from build123d import *

# Parameters (mm, degrees)
BOSS_EXTRUDE1_DEPTH      = 25
CUT_EXTRUDE4_START       = 8.5
CUT_EXTRUDE4_DEPTH       = 8
SKETCH10_R               = 4.2
CUT_EXTRUDE6_DEPTH       = 122.590026426
SKETCH11_W               = 24
SKETCH11_H               = 24.52
BOSS_EXTRUDE2_DEPTH      = 10
CUT_EXTRUDE7_DEPTH       = 122.590026426
CUT_EXTRUDE8_START       = 5.5
SKETCH14_W               = 24
SKETCH14_H               = 20.52
CUT_EXTRUDE8_DEPTH       = 2
SKETCH22_R               = 12.6
CUT_EXTRUDE16_DEPTH      = 122.590026426
SKETCH24_W               = 17.5
SKETCH24_H               = 12
BOSS_EXTRUDE3_DEPTH      = 25
FILLET6_R                = 15
FILLET7_R                = 1
SKETCH25_R               = 3
CUT_EXTRUDE18_DEPTH      = 25
SKETCH26_W               = 2.5
SKETCH26_H               = 20
CUT_EXTRUDE19_DEPTH      = 25
SHELL14_START            = 9.25
SHELL14_DEPTH            = 1.5
SHELL14_START_2          = 3
SHELL14_2_DEPTH          = 19
SHELL14_3_OUTLINE_R      = 9.2
SHELL14_3_DEPTH          = 0.5
SHELL14_START_3          = 21.5
SHELL14_4_OUTLINE_R      = 9.2
SHELL14_4_DEPTH          = 0.5
SHELL14_START_4          = 8
SHELL14_5_DEPTH          = 2.75
SHELL14_START_5          = 19.25
SHELL14_6_DEPTH          = 1.5
SKETCH27_W               = 17.72
SKETCH27_H               = 18.5
CUT_EXTRUDE20_DEPTH      = 10
SKETCH28_W               = 14
SKETCH28_H               = 35
CUT_EXTRUDE21_DEPTH      = 3
SKETCH29_W               = 14
SKETCH29_H               = 35
CUT_EXTRUDE22_DEPTH      = 3
FILLET8_R                = 4
FILLET9_R                = 4
FILLET10_R               = 1
CUT_EXTRUDE23_DEPTH      = 132.116752851
CUT_EXTRUDE23_DEPTH_BACK = 132.116752851
SKETCH32_W               = 24
SKETCH32_H               = 0.7
CUT_EXTRUDE24_DEPTH      = 132.116752851
FILLET11_R               = 3
BOSS_EXTRUDE4_REACH      = 133.117
SKETCH33_W               = 28
SKETCH33_H               = 2


with BuildPart() as part:
    # Sketch1 → Boss-Extrude1 (new body)
    with BuildSketch(Plane.XY):
        with BuildLine():
            Line((30, 0), (30, 75))
            ThreePointArc((30, 75), (15, 113.093476939), (0, 75))
            Line((0, 75), (0, 0))
            ThreePointArc((0, 0), (15, -15), (30, 0))
        make_face()
    extrude(amount=BOSS_EXTRUDE1_DEPTH)

    # Sketch9 → Cut-Extrude4 (cut)
    with BuildSketch(Plane.XY.offset(CUT_EXTRUDE4_START)):
        with BuildLine():
            Line((7.015640289, 0), (0, -3.844579475))
            Line((0, -3.844579475), (0, -19.136394538))
            Line((0, -19.136394538), (30, -19.136394538))
            Line((30, -19.136394538), (30, -3.844579475))
            Line((30, -3.844579475), (22.984359711, 0))
            ThreePointArc((22.984359711, 0), (15, 8.5), (7.015640289, 0))
        make_face()
    extrude(amount=CUT_EXTRUDE4_DEPTH, mode=Mode.SUBTRACT)

    # Sketch10 → Cut-Extrude6 (cut, through all)
    with BuildSketch(Plane.XY):
        with Locations(Location((15, 0.5, 0), (0, 0, 180))):
            Circle(SKETCH10_R)
    extrude(amount=CUT_EXTRUDE6_DEPTH, mode=Mode.SUBTRACT)

    # Sketch11 → Boss-Extrude2 (add)
    with BuildSketch(Plane(origin=(0, 0, 0), x_dir=(-1, 0, 0), z_dir=(0, 0, -1))):
        with Locations((-15, 32.26)):
            Rectangle(SKETCH11_W, SKETCH11_H)
    extrude(amount=BOSS_EXTRUDE2_DEPTH)

    # Sketch12 → Cut-Extrude7 (cut, through all)
    with BuildSketch(Plane(origin=(0, 0, 0), x_dir=(-1, 0, 0), z_dir=(0, 0, -1))):
        Polygon((-3, 42.52), (-3, 22), (-6.14, 23), (-23.86, 23), (-27, 22), (-27, 42.52), (-23.86, 41.52), (-6.14, 41.52), align=None)
    extrude(amount=CUT_EXTRUDE7_DEPTH, mode=Mode.SUBTRACT)

    # Sketch14 → Cut-Extrude8 (cut)
    with BuildSketch(Plane(origin=(0, 0, 0), x_dir=(-1, 0, 0), z_dir=(0, 0, -1)).offset(CUT_EXTRUDE8_START)):
        with Locations((-15, 32.26)):
            Rectangle(SKETCH14_W, SKETCH14_H)
    extrude(amount=CUT_EXTRUDE8_DEPTH, mode=Mode.SUBTRACT)

    # Sketch22 → Cut-Extrude16 (cut, through all)
    with BuildSketch(Plane.XY):
        with Locations((15, 91.093476939)):
            Circle(SKETCH22_R)
    extrude(amount=CUT_EXTRUDE16_DEPTH, mode=Mode.SUBTRACT)

    # Sketch24 → Boss-Extrude3 (add)
    with BuildSketch(Plane.XY):
        with Locations((15, 117.278558064)):
            Rectangle(SKETCH24_W, SKETCH24_H)
    extrude(amount=BOSS_EXTRUDE3_DEPTH)

    # Fillet6
    fillet6_edges = [part.edges().sort_by_distance(p)[0] for p in [
        (0, 75, 12.5),
        (30, 75, 12.5),
    ]]
    fillet(fillet6_edges, radius=FILLET6_R)

    # Fillet7
    fillet7_edges = [part.edges().sort_by_distance(p)[0] for p in [
        (6.25, 123.278558064, 12.5),
        (23.75, 123.278558064, 12.5),
    ]]
    fillet(fillet7_edges, radius=FILLET7_R)

    # Sketch25 → Cut-Extrude18 (cut)
    with BuildSketch(Plane(origin=(23.75, 0, 23.75), x_dir=(0, 0, 1), z_dir=(-1, 0, 0))):
        with Locations(Location((-11.25, 118.278558064, 0), (0, 0, 180))):
            Circle(SKETCH25_R)
    extrude(amount=CUT_EXTRUDE18_DEPTH, mode=Mode.SUBTRACT)

    # Sketch26 → Cut-Extrude19 (cut)
    with BuildSketch(Plane(origin=(0, 0, 0), x_dir=(-1, 0, 0), z_dir=(0, 0, -1))):
        with Locations((-15, 113.278558064)):
            Rectangle(SKETCH26_W, SKETCH26_H)
    extrude(amount=-CUT_EXTRUDE19_DEPTH, mode=Mode.SUBTRACT)

    # Shell14: read off the stored shape, not the designer's step
    # Shell14 outline → Shell14 (cut)
    with BuildSketch(Plane.YZ.offset(SHELL14_START)):
        with BuildLine():
            Line((118.278558064, 22), (113.278558064, 22))
            Line((113.278558064, 22), (113.278558064, 15.81662479))
            ThreePointArc((113.278558064, 15.81662479), (115.441283733, 17.786764074), (118.278558064, 18.5))
            Line((118.278558064, 18.5), (118.278558064, 22))
        make_face()
        with BuildLine():
            ThreePointArc((118.278558064, 6.5), (115.441283733, 7.213235926), (113.278558064, 9.18337521))
            Line((113.278558064, 9.18337521), (113.278558064, 3))
            Line((113.278558064, 3), (118.278558064, 3))
            Line((118.278558064, 3), (118.278558064, 6.5))
        make_face()
    extrude(amount=SHELL14_DEPTH, mode=Mode.SUBTRACT)

    # Shell14 2 outline → Shell14 2 (cut)
    with BuildSketch(Plane.XY.offset(SHELL14_START_2)):
        with BuildLine():
            Line((20.75, 113.278558064), (19.25, 113.278558064))
            Line((19.25, 113.278558064), (19.25, 106.10339033))
            ThreePointArc((19.25, 106.10339033), (15, 75.493476939), (10.75, 106.10339033))
            Line((10.75, 106.10339033), (10.75, 113.278558064))
            Line((10.75, 113.278558064), (9.25, 113.278558064))
            Line((9.25, 113.278558064), (9.25, 109.202521641))
            ThreePointArc((9.25, 109.202521641), (-3.041191716, 97.052956906), (-0.405405405, 79.972618866))
            ThreePointArc((-0.405405405, 79.972618866), (2.127502776, 74.973191279), (3, 69.437069112))
            Line((3, 69.437069112), (3, 3.500970796))
            Line((3, 3.500970796), (4.734171365, 4.451298829))
            ThreePointArc((4.734171365, 4.451298829), (15, 11.5), (25.265828635, 4.451298829))
            Line((25.265828635, 4.451298829), (27, 3.500970796))
            Line((27, 3.500970796), (27, 69.437069112))
            ThreePointArc((27, 69.437069112), (27.872497224, 74.973191279), (30.405405405, 79.972618866))
            ThreePointArc((30.405405405, 79.972618866), (33.041191716, 97.052956906), (20.75, 109.202521641))
            Line((20.75, 109.202521641), (20.75, 113.278558064))
        make_face()
    extrude(amount=SHELL14_2_DEPTH, mode=Mode.SUBTRACT)

    # Shell14 3 outline → Shell14 3 (cut)
    with BuildSketch(Plane.XY.offset(SHELL14_START_2)):
        with BuildLine():
            Line((27, 0), (27, 3.500970796))
            Line((27, 3.500970796), (25.265828635, 4.451298829))
            ThreePointArc((25.265828635, 4.451298829), (15, 11.5), (4.734171365, 4.451298829))
            Line((4.734171365, 4.451298829), (3, 3.500970796))
            Line((3, 3.500970796), (3, 0))
            ThreePointArc((3, 0), (15, -12), (27, 0))
        make_face()
        with Locations((15, 0.5)):
            Circle(SHELL14_3_OUTLINE_R, mode=Mode.SUBTRACT)
    extrude(amount=SHELL14_3_DEPTH, mode=Mode.SUBTRACT)

    # Shell14 4 outline → Shell14 4 (cut)
    with BuildSketch(Plane.XY.offset(SHELL14_START_3)):
        with BuildLine():
            Line((27, 0), (27, 3.500970796))
            Line((27, 3.500970796), (25.265828635, 4.451298829))
            ThreePointArc((25.265828635, 4.451298829), (15, 11.5), (4.734171365, 4.451298829))
            Line((4.734171365, 4.451298829), (3, 3.500970796))
            Line((3, 3.500970796), (3, 0))
            ThreePointArc((3, 0), (15, -12), (27, 0))
        make_face()
        with Locations((15, 0.5)):
            Circle(SHELL14_4_OUTLINE_R, mode=Mode.SUBTRACT)
    extrude(amount=SHELL14_4_DEPTH, mode=Mode.SUBTRACT)

    # Shell14 5 outline → Shell14 5 (add)
    with BuildSketch(Plane.YZ.offset(SHELL14_START_4)):
        with BuildLine():
            Line((113.278558064, 9.18337521), (113.278558064, 15.81662479))
            ThreePointArc((113.278558064, 15.81662479), (112.278558064, 12.5), (113.278558064, 9.18337521))
        make_face()
    extrude(amount=SHELL14_5_DEPTH)

    # Shell14 6 outline → Shell14 6 (add)
    with BuildSketch(Plane.YZ.offset(SHELL14_START_5)):
        with BuildLine():
            Line((113.278558064, 9.18337521), (113.278558064, 15.81662479))
            ThreePointArc((113.278558064, 15.81662479), (112.278558064, 12.5), (113.278558064, 9.18337521))
        make_face()
    extrude(amount=SHELL14_6_DEPTH)

    # Sketch27 → Cut-Extrude20 (cut)
    with BuildSketch(Plane(origin=(0, 0, 0), x_dir=(-1, 0, 0), z_dir=(0, 0, -1))):
        with Locations((-15, 32.25)):
            Rectangle(SKETCH27_W, SKETCH27_H)
    extrude(amount=-CUT_EXTRUDE20_DEPTH, mode=Mode.SUBTRACT)

    # Sketch28 → Cut-Extrude21 (cut)
    with BuildSketch(Plane.ZY):
        with Locations((12.5, 32.5)):
            Rectangle(SKETCH28_W, SKETCH28_H)
    extrude(amount=-CUT_EXTRUDE21_DEPTH, mode=Mode.SUBTRACT)

    # Sketch29 → Cut-Extrude22 (cut)
    with BuildSketch(Plane(origin=(30, 0, -30), x_dir=(0, 0, 1), z_dir=(-1, 0, 0))):
        with Locations((42.5, 32.5)):
            Rectangle(SKETCH29_W, SKETCH29_H)
    extrude(amount=CUT_EXTRUDE22_DEPTH, mode=Mode.SUBTRACT)

    # Fillet8
    fillet8_edges = [part.edges().sort_by_distance(p)[0] for p in [
        (1.5, 15, 19.5),
        (1.5, 50, 19.5),
        (1.5, 50, 5.5),
        (1.5, 15, 5.5),
        (28.5, 50, 5.5),
        (28.5, 15, 5.5),
        (28.5, 15, 19.5),
        (28.5, 50, 19.5),
    ]]
    fillet(fillet8_edges, radius=FILLET8_R)

    # Fillet9
    # the kernel refuses this fillet: 4 mm, written as the material it adds along each edge
    with BuildSketch(Plane(origin=(3, 3.500970796, 3.5), x_dir=(0, 1, 0), z_dir=(0, 0, 1))) as fillet9_piece_1:
        with BuildLine():
            CenterArc((4.246692788, -4), FILLET9_R, 90, 55.496459683)
            Line((0.950328033, -1.734171365), (0.884400738, -1.688854792))
            ThreePointArc((0.884400738, -1.688854792), (0.405007614, -0.905531477), (-0.070156403, -0.038445795))
            Line((-0.070156403, -0.038445795), (0, 0.08))
            Line((0, 0.08), (4.246692788, 0.08))
            Line((4.246692788, 0.08), (4.246692788, 0))
        make_face()
    extrude(amount=18)
    with BuildSketch(Plane(origin=(27, 3.500970796, 3.5), x_dir=(0, 1, 0), z_dir=(0, 0, 1))) as fillet9_piece_2:
        with BuildLine():
            CenterArc((4.246692788, 4), FILLET9_R, 214.503540317, 55.496459683)
            Line((0.950328033, 1.734171365), (0.884400738, 1.688854792))
            ThreePointArc((0.884400738, 1.688854792), (0.405007614, 0.905531477), (-0.070156403, 0.038445795))
            Line((-0.070156403, 0.038445795), (0, -0.08))
            Line((0, -0.08), (4.246692788, -0.08))
            Line((4.246692788, -0.08), (4.246692788, 0))
        make_face()
    extrude(amount=18)

    # Fillet10
    fillet10_edges = [part.edges().sort_by_distance(p)[0] for p in [
        (25.265828635, 4.451298829, 12.5),
        (4.734171365, 4.451298829, 12.5),
    ]]
    fillet(fillet10_edges, radius=FILLET10_R)

    # Sketch30 → Cut-Extrude23 (cut, two sides: drawn at the far end of the back side and taken through both)
    with BuildSketch(Plane(origin=(0, 0, 0), x_dir=(0, 0, -1), z_dir=(1, 0, 0)).offset(-CUT_EXTRUDE23_DEPTH_BACK)):
        Polygon((10, 42.52), (10, 41.52), (7.5, 41.52), (7.5, 42.12), align=None)
        Polygon((10, 22), (10, 23), (7.5, 23), (7.5, 22.4), align=None)
    extrude(amount=CUT_EXTRUDE23_DEPTH + CUT_EXTRUDE23_DEPTH_BACK, mode=Mode.SUBTRACT)

    # Sketch32 → Cut-Extrude24 (cut, through all)
    with BuildSketch(Plane(origin=(0, 0, 0), x_dir=(-1, 0, 0), z_dir=(0, 0, -1))):
        with Locations((-15, 44.17)):
            Rectangle(SKETCH32_W, SKETCH32_H)
        with Locations((-15, 20.35)):
            Rectangle(SKETCH32_W, SKETCH32_H)
    extrude(amount=CUT_EXTRUDE24_DEPTH, mode=Mode.SUBTRACT)

    # Fillet11
    fillet11_edges = [part.edges().sort_by_distance(p)[0] for p in [
        (15, 43.82, 0),
        (15, 20.7, 0),
    ]]
    fillet(fillet11_edges, radius=FILLET11_R)

    # Sketch33 → Boss-Extrude4 (add, up to next)
    with BuildSketch(Plane(origin=(0, 0, 0), x_dir=(-1, 0, 0), z_dir=(0, 0, -1)), mode=Mode.PRIVATE) as boss_extrude4_sk1:
        with Locations((-15, 71)):
            Rectangle(SKETCH33_W, SKETCH33_H)
    boss_extrude4_tool1 = extrude(boss_extrude4_sk1.sketch, amount=-BOSS_EXTRUDE4_REACH, mode=Mode.PRIVATE) - part.part
    add(boss_extrude4_tool1.solids().sort_by_distance((15, 71, 0))[0])


solid = part.part
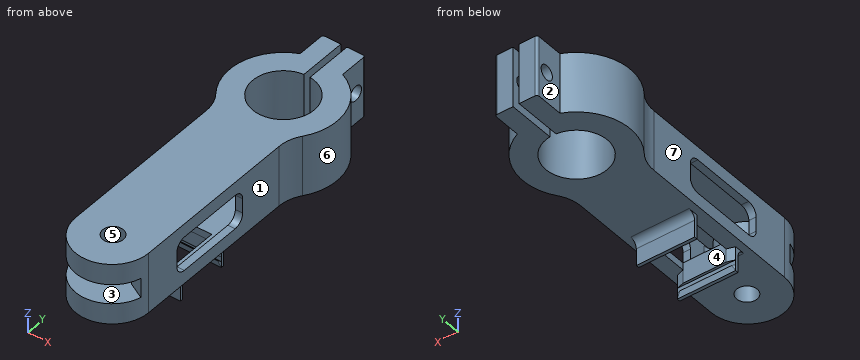
Geometry check sheet. Reference: the model listing, model coordinates, mm. Face numbers are marked on the shaded views. A direction names the side the tool comes from. Give positions to 0.01 mm unless a question says otherwise; leave off trailing zeros. Order: outer loops, then holes, each group sorted by start corner. A loop starts at its lowest first (then second) coordinate and runs counter-clockwise, first axis right, second up.
1. Sectioned sample at B-B (z = 12.5). State how many separate pieces and enclosed holes the cut face has, then the cut area to 3 significant figures.
Completed:
separate pieces: 4
enclosed holes: 1
area: 1,060 mm2
2. Sectioned sample at A-A (y = 31). Record the boundary of the cut face in (x, z).
Completed:
outline: (0, 0) - (6.14, 0) - (6.14, 3) - (3, 3) - (3, 5.5) - (0, 5.5) - close; (0, 19.5) - (3, 19.5) - (3, 22) - (27, 22) - (27, 19.5) - (30, 19.5) - (30, 25) - (0, 25) - close; (23.86, 0) - (30, 0) - (30, 5.5) - (27, 5.5) - (27, 3) - (23.86, 3) - close
3. Scan lines: line 1 (Y direction, x = 15, z = 6); line 2 (Y direction, x = 15, z = 13); line 3 (Y direction, x = 15, z = 2.25). Record each from-to range of solid material in increasing order.
Completed:
line 1: y = -15 to -3.7, 4.7 to 11.5, 70 to 72, 75.49 to 78.49
line 2: y = 8.5 to 11.5, 70 to 72, 75.49 to 78.49
line 3: y = -15 to -3.7, 4.7 to 23, 41.5 to 78.49
4. Draft check along Y on the marked faces 5, 6 and 7. Enter one of: pulls with the +Y half, pulls with the -Y half, needs draft (parallel to the pull), parting line crosses it, or undercut.
Completed:
face 5: undercut
face 6: parting line crosses it
face 7: needs draft
5. Access from +Z, -Z, +X, -X, +Y, -Y to the whole of each face (thin tool, end or side, straight path). Record for the marked faces 1, 2, 3 and 4.
Completed:
face 1: +Z, -Z, +X, -Y
face 2: +Z, -Z, -X, +Y
face 3: -Y
face 4: -Z
6. Depth check by flat-ended pin: pin 1 (22 mm diameter, centred on x = 6.5, y = 77.5, fed in from -Z); pin 2 (4.5 mm diameter, centred on y = 45.5, z = -3, fed in from +X); pin 3 (3 mm diameter, centred on x = -0.5, z = 16, fed in from +Y). Enter the tip coordinate at first touch or a pass-through.
Completed:
pin 1: stops at z = 0
pin 2: stops at x = 27
pin 3: stops at y = 108.06
